Can you work these out from the drawing? Everything is in mm from the part's minimum corner. Round coordinates to 2 decimals unless told otherwise and drop trailing zeros. Write each loop counter-clockwise with the first axis right and the second up, starting at its lowest first coordinate (ties: lowest second). Pieces come first, ordered by that corner, then holes. Notation, with made-up numbers: (27.5, 11.5) -> (50.5, 11.5) arc R17 ccw to (50.5, 42.5) -> close; hole circle Ø1 at (26.25, 47). An arc over 180 degrees is marked (long way). One line per question, with ' | ' between items. Start each with the question number.
1. If I drill on line 1 along Z through (x, y) = (60, 2.85); line 2 along X through (y, z) = (0.8, 25) (1 decimal); line 3 along Z through (x, y) = (16, 1.4), over which ranges is the centre line in solid material (lowest first)? Write a range as [from, to].
2. Imagine slicing it at C-C, the plane y = 1.3. List the corners of the cut face in (x, z) for me (1 decimal).
3. Imagine slicing it at B-B, the plane x = 34. List the corners of the cut face in (y, z) for me.
4. Imagine slicing it at A-A, the plane z = 17. List the corners of the cut face in (x, y) for me (1 decimal).
5. For pin 1 Ø3.5 at (x, z) = (60.02, 21.18) entering from -Y, with a flat end and sliding along its axis, tell me the tip position at first contact or that it passes through.
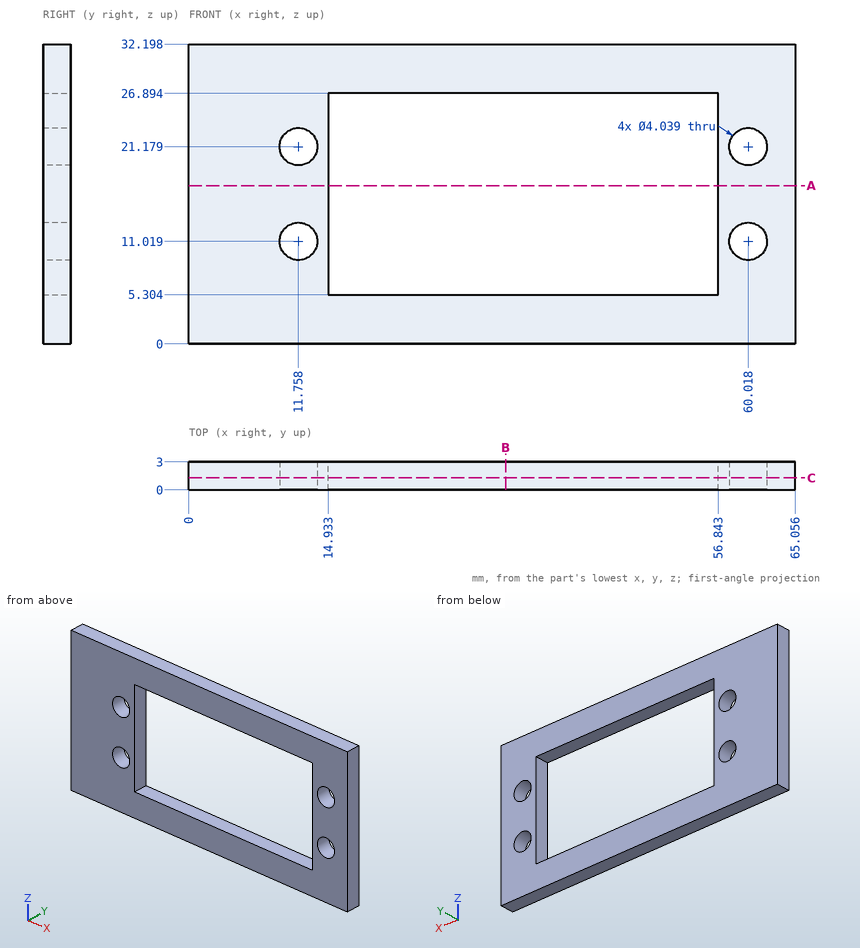
Geometry results:
1) line 1: z = [0, 9], [13.04, 19.16], [23.2, 32.2] | line 2: x = [0, 14.9], [56.8, 65.1] | line 3: z = [0, 5.3], [26.89, 32.2]
2) outline: (0, 0) -> (65.1, 0) -> (65.1, 32.2) -> (0, 32.2) -> close; hole circle Ø4 at (11.8, 11); hole circle Ø4 at (11.8, 21.2); hole (14.9, 5.3) -> (56.8, 5.3) -> (56.8, 26.9) -> (14.9, 26.9) -> close; hole circle Ø4 at (60, 11); hole circle Ø4 at (60, 21.2)
3) outline: (0, 0) -> (3, 0) -> (3, 5.3) -> (0, 5.3) -> close; (0, 26.89) -> (3, 26.89) -> (3, 32.2) -> (0, 32.2) -> close
4) outline: (0, 0) -> (14.9, 0) -> (14.9, 3) -> (0, 3) -> close; (56.8, 0) -> (65.1, 0) -> (65.1, 3) -> (56.8, 3) -> close
5) pin 1: passes through
